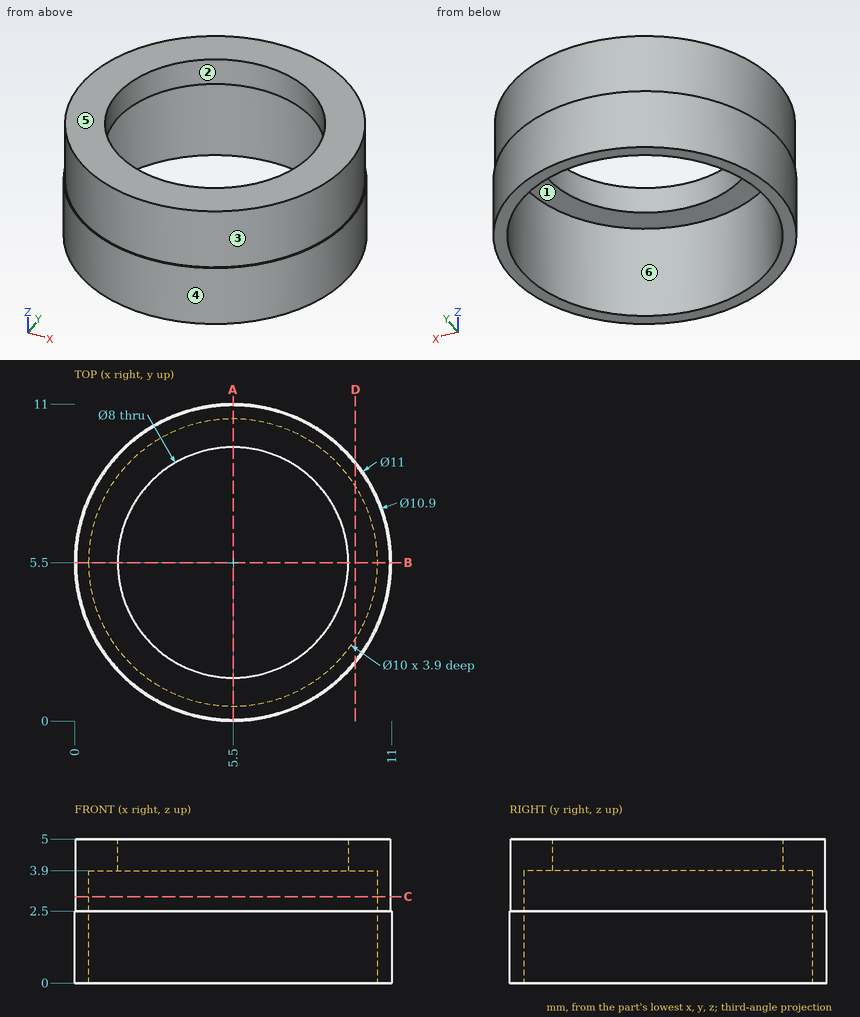
Source: three-view drawing plus pictorial views. Frame: mm from the lowest corner of the part. A direction names the side the tool comes from. Round coordinates to 2 decimals unless told otherwise and drop trailing zeros. Loops run counter-clockwise (first coordinate to the right, second up) from the corner with the lowest first, then second, coordinate; pieces in that order, holes last. Notation, with made-up numbers: (27.25, 18.25) -> (46.25, 18.25) arc R29 ccw to (46.25, 48.25) -> close; hole circle Ø10 at (21, 23). An arc over 180 degrees is marked (long way). Use one line per item in the form item = value.
Item 1: Contact query for flat-ended pins moving along their axis: pin 1 Ø2 at (y, z) = (4.5, 4.5) entering from -X; pin 2 Ø1.5 at (x, z) = (7, 3) entering from +Y. Output: stop coordinate, or through.
Evaluation:
pin_1 = 0.05
pin_2 = 10.92
Item 2: Cut plane C-C on z = 3. Output: boundary loops of the cut face in (x, y), then the cut area to 3 significant figures.
Evaluation:
outline = circle Ø10.9 at (5.5, 5.5); hole circle Ø10 at (5.5, 5.5)
area = 14.8 mm2
Item 3: Material intervals for probe 1 along Y at (x, z) = (5.5, 4.5); probe 2 along Y at (x, z) = (5.5, 2); probe 3 along X at (y, z) = (9.25, 1.4), sorted ascending.
Evaluation:
probe_1 = 0.05 to 1.5, 9.5 to 10.95
probe_2 = 0 to 0.5, 10.5 to 11
probe_3 = 1.48 to 2.19, 8.81 to 9.52
Item 4: Cut plane D-D on x = 9.75. Output: boundary loops of the cut face in (y, z), then the cut area to 3 significant figures.
Evaluation:
outline = (2.01, 0) -> (2.87, 0) -> (2.87, 3.9) -> (8.13, 3.9) -> (8.13, 0) -> (8.99, 0) -> (8.99, 2.5) -> (8.91, 2.5) -> (8.91, 5) -> (2.09, 5) -> (2.09, 2.5) -> (2.01, 2.5) -> close
area = 14.0 mm2
Item 5: Draft query along Y for the marked faces 4, 5 and 6. Return one class per face: released by +Y, released by -Y, zero draft, split by the parting line, or undercut.
Evaluation:
face_4 = split by the parting line
face_5 = zero draft
face_6 = undercut
Item 6: Access query for the marked faces 1, 2 and 3. Directions: +Z, -Z, +X, -X, +Y, -Y. A direction counts if a zero-diameter tool reaches every point of the face in a straight line with its end or side. Return the directions, or none.
Evaluation:
face_1 = -Z
face_2 = +Z, -Z
face_3 = +Z
Item 7: Cut plane A-A on x = 5.5. Output: boundary loops of the cut face in (y, z), then the cut area to 3 significant figures.
Evaluation:
outline = (0, 0) -> (0.5, 0) -> (0.5, 3.9) -> (1.5, 3.9) -> (1.5, 5) -> (0.05, 5) -> (0.05, 2.5) -> (0, 2.5) -> close; (9.5, 3.9) -> (10.5, 3.9) -> (10.5, 0) -> (11, 0) -> (11, 2.5) -> (10.95, 2.5) -> (10.95, 5) -> (9.5, 5) -> close
area = 6.95 mm2
